Geometry check sheet. Reference: the model listing, model coordinates, mm. Round coordinates to 2 decimals unless told otherwise and drop trailing zeros. Write each loop counter-clockwise with the first axis right and the second up, starting at its lowest first coordinate (ties: lowest second). Pieces come first, ordered by that corner, then holes. Notation, with made-up numbers: (-0.75, 17.5) - (46.25, 17.5) arc R20 cw to (46.25, 24.5) - close; hole circle Ø9 at (-16.5, 29.5). An arc over 180 degrees is marked (long way). Return JSON: item names as keys, results as strings. Group by question number.
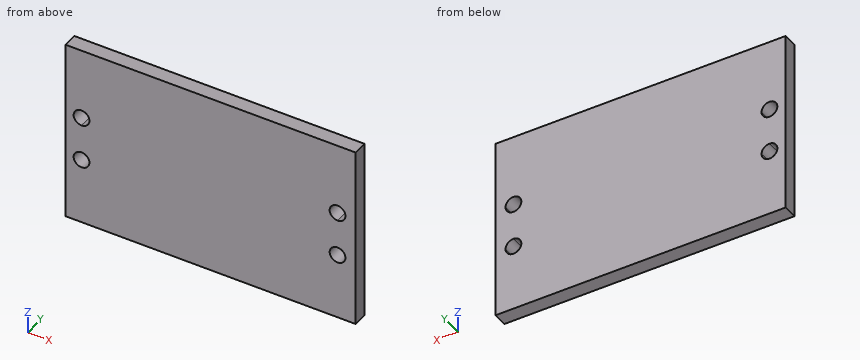
from build123d import *

# Parameters (mm, degrees)
F0_W     = 101.6
F0_H     = 63.5
F1_DEPTH = 5.08


with BuildPart() as f1:
    # F0 (on Front) → F1 (new body)
    with BuildSketch(Plane.XZ):
        with Locations((0.28524, 1.616135)):
            Rectangle(F0_W, F0_H)
        with BuildLine():
            ThreePointArc((-44.851955, -4.279891), (-42.894259, -5.090796), (-42.083355, -7.048491))
            ThreePointArc((-42.083355, -7.048491), (-46.809651, -9.006187), (-44.851955, -4.279891))
        make_face(mode=Mode.SUBTRACT)
        with BuildLine():
            ThreePointArc((44.758935, -4.285452), (46.712698, -5.094728), (47.521974, -7.048491))
            ThreePointArc((47.521974, -7.048491), (42.805171, -9.002255), (44.758935, -4.285452))
        make_face(mode=Mode.SUBTRACT)
        with BuildLine():
            ThreePointArc((-42.083355, 8.460924), (-42.894259, 6.503228), (-44.851955, 5.692324))
            ThreePointArc((-44.851955, 5.692324), (-46.809651, 10.41862), (-42.083355, 8.460924))
        make_face(mode=Mode.SUBTRACT)
        with BuildLine():
            ThreePointArc((47.527535, 8.460924), (46.71663, 6.503228), (44.758935, 5.692324))
            ThreePointArc((44.758935, 5.692324), (42.801239, 10.41862), (47.527535, 8.460924))
        make_face(mode=Mode.SUBTRACT)
    extrude(amount=F1_DEPTH)


solid = f1.part
1. Section check A-A (z = -6). Enter the section's corners in (x, y), and give its area (3 significant figures).
2. Depth check by flat-ended pin: pin 1 Ø5 at (x, z) = (44.76, -7.05) entering from +Y. Enter the tip coordinate at first touch or a pass-through.
3. Material ranges on line 1 along X through (y, z) = (-4.35, -6.5); line 2 along X through (y, z) = (-3, 11), recorded low to high.
Result sheet:
{
 "1": {"outline": "(-50.51, -5.08) - (-47.41, -5.08) - (-47.41, 0) - (-50.51, 0) - close; (-42.29, -5.08) - (42.2, -5.08) - (42.2, 0) - (-42.29, 0) - close; (47.32, -5.08) - (51.09, -5.08) - (51.09, 0) - (47.32, 0) - close", "area": "464 mm²"},
 "2": {"pin 1": "passes through"},
 "3": {"line 1": "x = -50.51 to -47.57, -42.14 to 42.05, 47.47 to 51.09", "line 2": "x = -50.51 to -45.96, -43.75 to 43.66, 45.86 to 51.09"}
}
